Source: CAD feature listing. Evaluate the final solid. Frame: model axes, mm. A direction names the side the tool comes from. Round coordinates to 2 decimals unless told otherwise and drop trailing zeros. Loops run counter-clockwise (first coordinate to the right, second up) from the corner with the lowest first, then second, coordinate; pieces in that order, holes last. Notation, with made-up numbers: M 29,0 L 84,0 A16 ccw 84,9 Z; hole C 11,-14.75 d2. An arc over 180 degrees is marked long. Answer as a JSON object with one key per item and string values.
from build123d import *

# Parameters (mm, degrees)
BOSS_EXTRUDE2_DEPTH = 55
SKETCH7_R           = 12.55
CUT_EXTRUDE2_DEPTH  = 64.969298353
SKETCH8_R           = 1.6
CUT_EXTRUDE3_DEPTH  = 72.1238248
SKETCH10_R          = 1.6
CUT_EXTRUDE5_DEPTH  = 8
SKETCH11_W          = 36.155443868
SKETCH11_H          = 8
CUT_EXTRUDE6_DEPTH  = 64.96929848
FILLET1_R           = 10


with BuildPart() as part:
    # Sketch4 → Boss-Extrude2 (new body)
    with BuildSketch(Plane(origin=(0, 0, 0), x_dir=(1, 0, 0), z_dir=(0, 1, 0))):
        with BuildLine():
            Line((-19.671845121, 26.078528358), (19.671845121, 26.078528358))
            Line((19.671845121, 26.078528358), (19.671845121, 12.578528358))
            ThreePointArc((19.671845121, 12.578528358), (14.48082404, 7.360388375), (14.5, 0))
            ThreePointArc((14.5, 0), (0, -14.5), (-14.5, 0))
            ThreePointArc((-14.5, 0), (-14.48082404, 7.360388375), (-19.671845121, 12.578528358))
            Line((-19.671845121, 12.578528358), (-19.671845121, 26.078528358))
        make_face()
    extrude(amount=BOSS_EXTRUDE2_DEPTH)

    # Sketch7 → Cut-Extrude2 (cut, through all)
    with BuildSketch(Plane(origin=(0, 0, 0), x_dir=(1, 0, 0), z_dir=(0, 1, 0))):
        with Locations(Location((0, 0, 0), (0, 0, 270))):
            Circle(SKETCH7_R)
    extrude(amount=CUT_EXTRUDE2_DEPTH, mode=Mode.SUBTRACT)

    # Sketch8 → Cut-Extrude3 (cut, through all)
    with BuildSketch(Plane(origin=(0, 0, -26.078528358), x_dir=(-1, 0, 0), z_dir=(0, 0, -1))):
        with Locations((0, 27.5)):
            Circle(SKETCH8_R)
    extrude(amount=-CUT_EXTRUDE3_DEPTH, mode=Mode.SUBTRACT)

    # Sketch10 → Cut-Extrude5 (cut)
    with BuildSketch(Plane(origin=(0, 0, -26.078528358), x_dir=(-1, 0, 0), z_dir=(0, 0, -1))):
        with Locations((8.838834765, 18.661165235)):
            Circle(SKETCH10_R)
        with Locations((8.838834765, 36.338834765)):
            Circle(SKETCH10_R)
        with Locations((-8.838834765, 36.338834765)):
            Circle(SKETCH10_R)
        with Locations((-8.838834765, 18.661165235)):
            Circle(SKETCH10_R)
    extrude(amount=-CUT_EXTRUDE5_DEPTH, mode=Mode.SUBTRACT)

    # Sketch11 → Cut-Extrude6 (cut, through all)
    with BuildSketch(Plane(origin=(0, 55, 0), x_dir=(1, 0, 0), z_dir=(0, 1, 0))):
        with Locations((0, 19.078528358)):
            Rectangle(SKETCH11_W, SKETCH11_H)
    extrude(amount=-CUT_EXTRUDE6_DEPTH, mode=Mode.SUBTRACT)

    # Fillet1
    fillet1_edges = [part.edges().sort_by_distance(p)[0] for p in [
        (14.5, 27.5, 0),
        (-14.5, 27.5, 0),
    ]]
    fillet(fillet1_edges, radius=FILLET1_R)


solid = part.part
Item 1: Section C-C on y = 23.5. Give the number of separate pieces and of enclosed holes in the cut face, then the cut area to 3 significant figures.
Answer sheet:
{"separate pieces": "1", "enclosed holes": "2", "area": "454 mm²"}
Item 2: Line query: probe 1 along X at (y, z) = (48.5, -16.5); probe 2 along Z at (x, y) = (16.5, 35); probe 3 along Y at (x, z) = (0, 13.9). Output: solid intervals per line, ascending. Write a range as from..to.
Answer sheet:
{"probe 1": "x = -19.67..-18.08, 18.08..19.67", "probe 2": "z = -26.08..-23.08, -15.08..-10.43", "probe 3": "y = 0..25.9, 29.1..55"}
Item 3: Pull-direction query (X, two-part tool) for faces 4 (the cylindrical face through (14.817, 27.115, -8.09)), 5 (the flat face through (18.078, 28, -19)), 6 (the flat face through (2, 55, -13)); classes: pulls with the +X half, pulls with the -X half, needs draft (parallel to the pull), parting line crosses it, or undercut.
Answer sheet:
{"face 4": "pulls with the +X half", "face 5": "undercut", "face 6": "needs draft"}
Item 4: Contact query for flat-ended pins moving along their axis: pin 1 Ø3 at (y, z) = (44.5, -6) entering from -X; pin 2 Ø3 at (y, z) = (26.5, -8) entering from -X; pin 3 Ø3 at (x, y) = (-8.84, 18.66) entering from -Z. Output: stop coordinate, or through.
Answer sheet:
{"pin 1": "stops at x = -14.54", "pin 2": "stops at x = -15.7", "pin 3": "stops at z = -15.08"}
Item 5: Section A-A on z = 8.5. Return the cut outline in (x, y), then the cut area to 3 significant figures.
Answer sheet:
{"outline": "M -11.75,0 L -9.23,0 L -9.23,55 L -11.75,55 Z; M 9.23,0 L 11.75,0 L 11.75,55 L 9.23,55 Z", "area": "277 mm²"}
Item 6: Section B-B on x = 0. Return the cut outline in (y, z).
Answer sheet:
{"outline": "M 0,-26.08 L 25.9,-26.08 L 25.9,-23.08 L 0,-23.08 Z; M 0,-15.08 L 25.9,-15.08 L 25.9,-12.55 L 0,-12.55 Z; M 0,12.55 L 25.9,12.55 L 25.9,14.5 L 0,14.5 Z; M 29.1,-26.08 L 55,-26.08 L 55,-23.08 L 29.1,-23.08 Z; M 29.1,-15.08 L 55,-15.08 L 55,-12.55 L 29.1,-12.55 Z; M 29.1,12.55 L 55,12.55 L 55,14.5 L 29.1,14.5 Z"}
Item 7: Access query for faces 1 (the flat face through (-18.078, 28, -19)), 2 (the flat face through (2, 0, -13)), 3 (the cylindrical face through (-8.631, 20.248, -24.6)). Directions: +Z, -Z, +X, -X, +Y, -Y. A direction counts if a zero-diameter tool reaches every point of the face in a straight line with its end or side. Return the directions, or none.
Answer sheet:
{"face 1": "+Y, -Y", "face 2": "+Z, -Z, +X, -X, -Y", "face 3": "-Z"}
